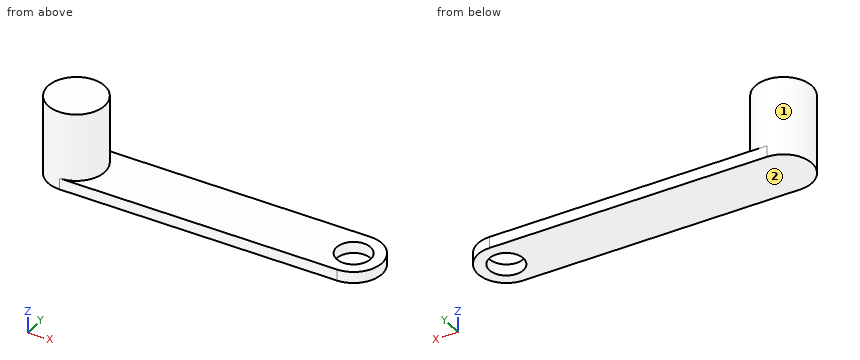
Autodesk Inventor part; units mm, degrees
ref_plane "YZ Plane" through (0, 0, 0) normal (1, 0, 0) x (0, 1, 0)
ref_plane "XZ Plane" through (0, 0, 0) normal (0, 1, 0) x (-1, 0, 0)
ref_plane "XY Plane" through (0, 0, 0) normal (0, 0, 1) x (1, 0, 0)
sketch "Boceto1" plane through (0, 0, 0) normal (0, 0, 1) x (1, 0, 0)
  line L0 (-4.4214, -2.4997) -> (115.5786, -2.4997) construction
  line L1 (-4.4214, -14.9997) -> (115.5786, -14.9997)
  line L2 (115.5786, 10.0003) -> (-4.4214, 10.0003)
  arc A0 (-4.4214, 10.0003) -> (-4.4214, -14.9997) centre (-4.4214, -2.4997) ccw
  arc A1 (115.5786, -14.9997) -> (115.5786, 10.0003) centre (115.5786, -2.4997) ccw
  circle A2 centre (115.5786, -2.4997) radius 7.5
  point P0 (0, 0)
  point P1 (55.5786, -2.4997)
  dimension "d3" = 120
  dimension "d4" = 25
  dimension "d5" = 15
extrude "Extrusión1" add sketch "Boceto1" along normal blind 5
sketch "Boceto4" plane through (0, 0, 5) normal (0, 0, 1) x (1, 0, 0)
  arc A0 (-4.4214, 10.0003) -> (-4.4214, -14.9997) centre (-4.4214, -2.4997) ccw
  circle A1 centre (-4.4214, -2.4997) radius 12.5
  point P0 (0, 0)
  point P1 (-4.4214, -14.9997)
  dimension "d12" = 25
extrude "Extrusión3" add sketch "Boceto4" along normal blind 30
properties part number "L1" material "Aluminio 6061"
Source: CAD feature listing. Evaluate the final solid. Frame: model axes, mm. Face numbers are marked on the shaded views. A direction names the side the tool comes from. Give positions to 0.01 mm unless a question says otherwise; leave off trailing zeros. Loops run counter-clockwise (first coordinate to the right, second up) from the corner with the lowest first, then second, coordinate; pieces in that order, holes last. Notation, with made-up numbers: (38.25, -7) -> (55.25, -7) arc R22 ccw to (55.25, 13) -> close; hole circle Ø5 at (-14.75, 46). An arc over 180 degrees is marked (long way). Use a Markdown table: item, result. Add a question column.
(1) Access query for the marked faces 1 and 2. Directions: +Z, -Z, +X, -X, +Y, -Y. A direction counts if a zero-diameter tool reaches every point of the face in a straight line with its end or side. Return the directions, or none.
(2) Section query C-C (y = 7). Output: boundary loops of the cut face in (x, z), then the cut area to 3 significant figures.
(3) Section query D-D (z = 28). Output: boundary loops of the cut face in (x, y).
(4) Ray query, line 1 (Z direction, x = 95, y = -7.75); line 2 (X direction, y = -2.5, z = 26.5); line 3 (X direction, y = 5.75, z = 13). Return the intervals inside material, ascending.
(5) Section query A-A (y = -8). Output: boundary loops of the cut face in (x, z).
(6) First-contact query: pin 1 Ø10 at (y, z) = (0, 23.5) entering from -X; pin 2 Ø4 at (y, z) = (1, 26) entering from -X. Flat tips, straight axial feed; report the tip coordinate or a pass-through.
(7) Section query B-B (x = 75). Output: boundary loops of the cut face in (y, z).
Checked values:
| question | item | result |
|---|---|---|
| 1 | face 1 | +Z |
| 1 | face 2 | -Z, +X, -X, +Y, -Y |
| 2 | outline | (-12.55, 0) -> (123.7, 0) -> (123.7, 5) -> (3.7, 5) -> (3.7, 35) -> (-12.55, 35) -> close |
| 2 | area | 1,170 mm^2 |
| 3 | outline | circle Ø25 at (-4.42, -2.5) |
| 4 | line 1 | 0 to 5 |
| 4 | line 2 | -16.92 to 8.08 |
| 4 | line 3 | -13.81 to 4.97 |
| 5 | outline | (-15.65, 0) -> (110.48, 0) -> (110.48, 5) -> (6.8, 5) -> (6.8, 35) -> (-15.65, 35) -> close; (120.68, 0) -> (126.8, 0) -> (126.8, 5) -> (120.68, 5) -> close |
| 6 | pin 1 | x = -16.92 |
| 6 | pin 2 | x = -16.83 |
| 7 | outline | (-15, 0) -> (10, 0) -> (10, 5) -> (-15, 5) -> close |
